Read the model definition and answer for the solid it produces. Units are mm, in the model's axes. A direction names the side the tool comes from. Coordinates: 2 decimals unless noted, no trailing zeros. Write each loop counter-clockwise with the first axis right and the second up, starting at its lowest first coordinate (ties: lowest second). Pieces come first, ordered by that corner, then holes. Notation, with made-up numbers: (78, 61.5) -> (96, 61.5) arc R17 ccw to (96, 65.5) -> close; hole circle Ø6 at (-1, 79). An arc over 180 degrees is marked (long way). Use CSV: the item, a comma, the result in double quotes.
from build123d import *

# Parameters (mm, degrees)
SKETCH1_R               = 50
BOSS_EXTRUDE1_DEPTH     = 5
BOSS_EXTRUDE3_START     = 5
BOSS_EXTRUDE3_DEPTH     = 5
DRAFT2_ANGLE            = -45
CUT_EXTRUDE3_DEPTH      = 72.414284285
CUT_EXTRUDE3_DEPTH_BACK = 72.414284285
SKETCH3_R               = 7.5
CUT_EXTRUDE5_START      = -6.666666667
CUT_EXTRUDE5_DEPTH      = 6.666666667
SKETCH5_R               = 3.55
SKETCH5_R_2             = 1.55
CUT_EXTRUDE6_DEPTH      = 72.414284285
SKETCH5_3_R             = 3.55
SKETCH5_3_R_2           = 1.55
BOSS_EXTRUDE4_DEPTH     = 2.5
CUT_EXTRUDE8_DEPTH      = 72.414284285
CHAMFER1_SIZE           = 5


with BuildPart() as part:
    # Sketch1 → Boss-Extrude1 (new body)
    with BuildSketch(Plane(origin=(0, 0, 0), x_dir=(1, 0, 0), z_dir=(0, 1, 0))):
        with Locations(Location((0, 0, 0), (0, 0, 270))):
            Circle(SKETCH1_R)
    extrude(amount=-BOSS_EXTRUDE1_DEPTH)

    # Sketch1<6> → Boss-Extrude3 (add)
    with BuildSketch(Plane(origin=(0, 0, 0), x_dir=(1, 0, 0), z_dir=(0, 1, 0)).offset(BOSS_EXTRUDE3_START)):
        with BuildLine():
            Line((-24.148145658, 6.470476128), (-34.10533906, -36.562629112))
            ThreePointArc((-34.10533906, -36.562629112), (0, -50), (34.10533906, -36.562629112))
            Line((34.10533906, -36.562629112), (24.148145658, 6.470476128))
            Line((24.148145658, 6.470476128), (12.940952256, 48.296291314))
            ThreePointArc((12.940952256, 48.296291314), (0, 50), (-12.940952256, 48.296291314))
            Line((-12.940952256, 48.296291314), (-24.148145658, 6.470476128))
        make_face()
    extrude(amount=-BOSS_EXTRUDE3_DEPTH)

    # Draft2
    draft2_faces = [part.faces().sort_by_distance(p)[0] for p in [
        (-29.126742359, 2.5, 15.046076492),
        (-18.544548957, 2.5, -27.383383721),
        (18.544548957, 2.5, -27.383383721),
        (29.126742359, 2.5, 15.046076492),
    ]]
    draft(draft2_faces, Plane.ZX, DRAFT2_ANGLE)

    # Sketch3 → Cut-Extrude3 (cut, two sides: drawn at the far end of the back side and taken through both)
    with BuildSketch(Plane.XZ.offset(5).offset(-CUT_EXTRUDE3_DEPTH_BACK)):
        with Locations(Location((0, 35.355339059, 0), (0, 0, 270))):
            Circle(SKETCH3_R)
    extrude(amount=CUT_EXTRUDE3_DEPTH + CUT_EXTRUDE3_DEPTH_BACK, mode=Mode.SUBTRACT)

    # Sketch4 → Cut-Extrude5 (cut)
    with BuildSketch(Plane.XZ.offset(5).offset(CUT_EXTRUDE5_START)):
        with BuildLine():
            ThreePointArc((18.178606224, 46.578302628), (0, 50), (-18.178606224, 46.578302628))
            Line((-18.178606224, 46.578302628), (-11.548494202, 30.571796264))
            ThreePointArc((-11.548494202, 30.571796264), (3.3e-08, 22.855339059), (11.548494227, 30.571796326))
            Line((11.548494227, 30.571796326), (18.178606224, 46.578302628))
        make_face()
    extrude(amount=CUT_EXTRUDE5_DEPTH, mode=Mode.SUBTRACT)

    # Sketch5 → Cut-Extrude6 (cut, through all)
    # profile 1 of 8: a face of its own
    with BuildSketch(Plane.XZ.offset(5)):
        with Locations(Location((25.355339059, 25.355339059, 0), (0, 0, 270))):
            Circle(SKETCH5_R)
        with Locations((25.355339059, 25.355339059)):
            Circle(SKETCH5_R_2, mode=Mode.SUBTRACT)
    # profile 2 of 8: a face of its own
    with BuildSketch(Plane.XZ.offset(5)):
        with Locations((25.355339059, 25.355339059)):
            Circle(SKETCH5_R_2)
    # profile 3 of 8: a face of its own
    with BuildSketch(Plane.XZ.offset(5)):
        with Locations(Location((25.355339059, -25.355339059, 0), (0, 0, 270))):
            Circle(SKETCH5_R)
        with Locations((25.355339059, -25.355339059)):
            Circle(SKETCH5_R_2, mode=Mode.SUBTRACT)
    # profile 4 of 8: a face of its own
    with BuildSketch(Plane.XZ.offset(5)):
        with Locations((25.355339059, -25.355339059)):
            Circle(SKETCH5_R_2)
    # profile 5 of 8: a face of its own
    with BuildSketch(Plane.XZ.offset(5)):
        with Locations(Location((-25.355339059, -25.355339059, 0), (0, 0, 270))):
            Circle(SKETCH5_R)
        with Locations((-25.355339059, -25.355339059)):
            Circle(SKETCH5_R_2, mode=Mode.SUBTRACT)
    # profile 6 of 8: a face of its own
    with BuildSketch(Plane.XZ.offset(5)):
        with Locations((-25.355339059, -25.355339059)):
            Circle(SKETCH5_R_2)
    # profile 7 of 8: a face of its own
    with BuildSketch(Plane.XZ.offset(5)):
        with Locations(Location((-25.355339059, 25.355339059, 0), (0, 0, 270))):
            Circle(SKETCH5_R)
        with Locations((-25.355339059, 25.355339059)):
            Circle(SKETCH5_R_2, mode=Mode.SUBTRACT)
    # profile 8 of 8: a face of its own
    with BuildSketch(Plane.XZ.offset(5)):
        with Locations((-25.355339059, 25.355339059)):
            Circle(SKETCH5_R_2)
    extrude(amount=-CUT_EXTRUDE6_DEPTH, mode=Mode.SUBTRACT)

    # Sketch5<3> → Boss-Extrude4 (add)
    # profile 1 of 4: a face of its own
    with BuildSketch(Plane.XZ.offset(5)):
        with Locations(Location((25.355339059, -25.355339059, 0), (0, 0, 270))):
            Circle(SKETCH5_3_R)
        with Locations(Location((25.355339059, -25.355339059, 0), (0, 0, 270))):
            Circle(SKETCH5_3_R_2, mode=Mode.SUBTRACT)
    # profile 2 of 4: a face of its own
    with BuildSketch(Plane.XZ.offset(5)):
        with Locations(Location((-25.355339059, -25.355339059, 0), (0, 0, 270))):
            Circle(SKETCH5_3_R)
        with Locations(Location((-25.355339059, -25.355339059, 0), (0, 0, 270))):
            Circle(SKETCH5_3_R_2, mode=Mode.SUBTRACT)
    # profile 3 of 4: a face of its own
    with BuildSketch(Plane.XZ.offset(5)):
        with Locations(Location((25.355339059, 25.355339059, 0), (0, 0, 270))):
            Circle(SKETCH5_3_R)
        with Locations(Location((25.355339059, 25.355339059, 0), (0, 0, 270))):
            Circle(SKETCH5_3_R_2, mode=Mode.SUBTRACT)
    # profile 4 of 4: a face of its own
    with BuildSketch(Plane.XZ.offset(5)):
        with Locations(Location((-25.355339059, 25.355339059, 0), (0, 0, 270))):
            Circle(SKETCH5_3_R)
        with Locations(Location((-25.355339059, 25.355339059, 0), (0, 0, 270))):
            Circle(SKETCH5_3_R_2, mode=Mode.SUBTRACT)
    extrude(amount=-BOSS_EXTRUDE4_DEPTH)

    # Sketch6 → Cut-Extrude8 (cut, through all)
    with BuildSketch(Plane(origin=(0, 5, 0), x_dir=(1, 0, 0), z_dir=(0, 1, 0))):
        with BuildLine():
            ThreePointArc((-0.574925376, -22.523405739), (0, -22.191472419), (0.574925376, -22.523405739))
            Line((0.574925376, -22.523405739), (19.793304237, -11.42766953))
            Line((19.793304237, -11.42766953), (19.793304237, 11.42766953))
            Line((19.793304237, 11.42766953), (0, 22.855339059))
            Line((0, 22.855339059), (-19.793304237, 11.42766953))
            Line((-19.793304237, 11.42766953), (-19.793304237, -11.42766953))
            Line((-19.793304237, -11.42766953), (-0.574925376, -22.523405739))
        make_face()
    extrude(amount=-CUT_EXTRUDE8_DEPTH, mode=Mode.SUBTRACT)

    # Chamfer1
    chamfer1_edges = [part.edges().sort_by_distance(p)[0] for p in [
        (-25.355339059, 5, 28.905339059),
        (25.355339059, 5, 28.905339059),
    ]]
    chamfer(chamfer1_edges, length=CHAMFER1_SIZE)


solid = part.part
1. A cutting plane is placed at C-C (z = -33). Give the vertices of the cut face in (x, y).
Solutions:
outline,"(-37.56, -5) -> (37.56, -5) -> (37.56, 0) -> (17.04, 0) -> (22.22, 5) -> (-22.22, 5) -> (-17.04, 0) -> (-37.56, 0) -> close"
2. For a pull along X with two mould halves and no side action, classify faces 5 (the flat face through (-9, 5, 22)), 6 (the cylindrical face through (-23, -1.3, -22.7)), 7 (the cylindrical face through (-21.91, 4.01, -24.5)) as pulls with the +X half, pulls with the -X half, needs draft (parallel to the pull), parting line crosses it, or undercut.
Solutions:
face 5,"needs draft"
face 6,"undercut"
face 7,"pulls with the -X half"
3. Find the intervals of material crossed by line 1 along Z through (x, y) = (6, 2.75); line 2 along X through (y, z) = (-2.25, 28); line 3 along Y through (x, z) = (-36.5, 15.5), in increasing order.
Solutions:
line 1,"z = -49.64 to -19.39, 19.39 to 30.86, 39.86 to 49.64"
line 2,"x = -41.42 to -27.72, -22.99 to -10.11, 10.11 to 22.99, 27.72 to 41.42"
line 3,"y = -5 to 0"
4. A cutting plane is placed at D-D (z = 3.5). Give the vertices of the cut face in (x, y).
Solutions:
outline,"(-49.88, -5) -> (-19.79, -5) -> (-19.79, 5) -> (-31.59, 5) -> (-26.46, 0) -> (-49.88, 0) -> close; (19.79, -5) -> (49.88, -5) -> (49.88, 0) -> (26.46, 0) -> (31.59, 5) -> (19.79, 5) -> close"
5. A cutting plane is placed at B-B (y = -1.25). Give the vertices of the cut face in (x, z), and give its area (3 significant figures).
Solutions:
outline,"(-18.18, 46.58) arc R50 ccw (long way) to (18.18, 46.58) -> (11.55, 30.57) arc R12.5 cw to (-11.55, 30.57) -> close; hole circle Ø7.1 at (-25.36, -25.36); hole circle Ø7.1 at (-25.36, 25.36); hole (-19.79, -11.43) -> (0, -22.86) -> (19.79, -11.43) -> (19.79, 11.43) -> (0.57, 22.52) arc R0.66 cw to (-0.57, 22.52) -> (-19.79, 11.43) -> close; hole circle Ø7.1 at (25.36, -25.36); hole circle Ø7.1 at (25.36, 25.36)"
area,"5,650 mm^2"
6. A tool of negligible diameter and unlimited length cuts with its end or side. For faces 1 (the flat face through (10.05, 0.07, 17.053)), 2 (the flat face through (-10, -5, -22)), 3 (the flat face through (-26.9, -2.5, 24.6)), 4 (the cylindrical face through (-0.206, -1.62, 22.857)), from which of +Z, -Z, +X, -X, +Y, -Y can it reach the whole face along a straight path? Write none if from no direction.
Solutions:
face 1,"+Y, -Y"
face 2,"+Z, -Z, +X, -X, -Y"
face 3,"+Y"
face 4,"+Z, -Y"
7. A cutting plane is placed at A-A (z = 14.5). Give the vertices of the cut face in (x, y).
Solutions:
outline,"(-47.85, -5) -> (-14.47, -5) -> (-14.47, 5) -> (-34.13, 5) -> (-29, 0) -> (-47.85, 0) -> close; (14.47, -5) -> (47.85, -5) -> (47.85, 0) -> (29, 0) -> (34.13, 5) -> (14.47, 5) -> close"
8. Each of these flat-tipped pins is pushed along its axis until it touches: pin 1 Ø2 at (x, z) = (28.5, -15.5) entering from +Y; pin 2 Ø3 at (y, z) = (-2, -1) entering from -X; pin 3 Ø6.5 at (x, z) = (25.36, 25.36) entering from +Y; pin 4 Ø3 at (x, z) = (25.36, 25.36) entering from +Y. Where does it stop, or does it pass through?
Solutions:
pin 1,"stops at y = 0"
pin 2,"stops at x = -50"
pin 3,"stops at y = -2.5"
pin 4,"passes through"
